Read the model definition and answer for the solid it produces. Units are mm, in the model's axes. Face numbers are marked on the shaded views. A direction names the side the tool comes from. Give positions to 0.01 mm unless a question says otherwise; leave off trailing zeros. Order: outer loops, then holes, each group sorted by start corner. A loop starts at its lowest first (then second) coordinate and runs counter-clockwise, first axis right, second up.
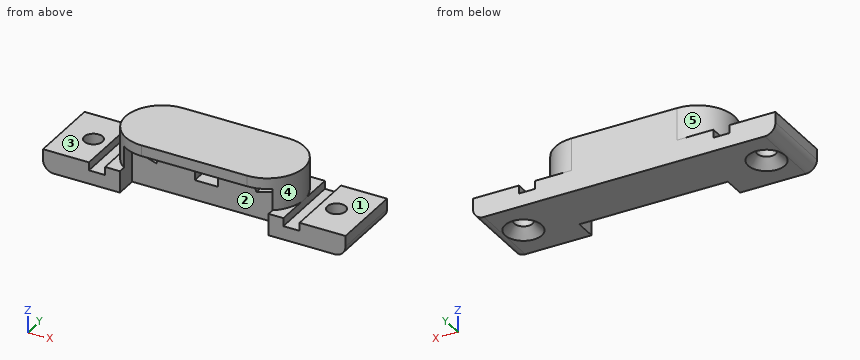
```python
from build123d import *

# Parameters (mm, degrees)
SKETCH_W        = 56
SKETCH_H        = 13.6
SKETCH_R        = 1.7
PAD_DEPTH       = 4
PAD001_DEPTH    = 6
SKETCH002_W     = 4.3
SKETCH002_H     = 1.7
POCKET_DEPTH    = 10
SKETCH003_W     = 27.5
SKETCH003_H     = 8.7
POCKET001_DEPTH = 4
SKETCH004_W     = 3
SKETCH004_H     = 1.5
POCKET002_DEPTH = 130.578947
CHAMFER_SIZE    = 1.7
CHAMFER001_SIZE = 1.7
FILLET_R        = 2
FILLET001_R     = 2


with BuildPart() as part:
    # Sketch → Pad (new body)
    with BuildSketch(Plane.XY):
        Rectangle(SKETCH_W, SKETCH_H)
        with Locations((-22.5, 0)):
            Circle(SKETCH_R, mode=Mode.SUBTRACT)
        with Locations((22.5, 0)):
            Circle(SKETCH_R, mode=Mode.SUBTRACT)
    extrude(amount=-PAD_DEPTH)

    # Sketch001 → Pad001 (new body)
    with BuildSketch(Plane.XY):
        with BuildLine():
            ThreePointArc((-9.75, 6.8), (-16.55, 0), (-9.75, -6.8))
            Line((-9.75, -6.8), (9.75, -6.8))
            ThreePointArc((9.75, -6.8), (16.55, 0), (9.75, 6.8))
            Line((-9.75, 6.8), (9.75, 6.8))
        make_face()
    extrude(amount=PAD001_DEPTH)

    # Sketch002 → Pocket (cut)
    with BuildSketch(Plane.XZ.offset(6.8)):
        Polygon((-12.857344, 3.612012), (-8.748385, 2.344555), (-9.249472, 0.720082), (-13.358432, 1.98754), align=None)
        with Locations((0, 0.5)):
            Rectangle(SKETCH002_W, SKETCH002_H)
        Polygon((8.748385, 2.344555), (12.857344, 3.612012), (13.358432, 1.98754), (9.249472, 0.720082), align=None)
    extrude(amount=-POCKET_DEPTH, mode=Mode.SUBTRACT)

    # Sketch003 → Pocket001 (cut)
    with BuildSketch(Plane.XZ.offset(6.8)):
        with Locations((0, -0.35)):
            Rectangle(SKETCH003_W, SKETCH003_H)
    extrude(amount=-POCKET001_DEPTH, mode=Mode.SUBTRACT)

    # Sketch004 → Pocket002 (cut, through all)
    with BuildSketch(Plane.XZ.offset(6.8)):
        with Locations((-18, -0.75)):
            Rectangle(SKETCH004_W, SKETCH004_H)
    pocket002 = extrude(amount=-POCKET002_DEPTH, mode=Mode.SUBTRACT)

    # Mirrored: Pocket002 across Sketch004 V_Axis
    add(pocket002.mirror(Plane(origin=(0, -6.8, 0), x_dir=(0, -1, 0), z_dir=(1, 0, 0))), mode=Mode.SUBTRACT)

    # Chamfer
    chamfer_edges = [part.edges().sort_by_distance(p)[0] for p in [
        (-24.2, 0, -4),
    ]]
    chamfer(chamfer_edges, length=CHAMFER_SIZE)

    # Chamfer001
    chamfer001_edges = [part.edges().sort_by_distance(p)[0] for p in [
        (20.8, 0, -4),
    ]]
    chamfer(chamfer001_edges, length=CHAMFER001_SIZE)

    # Fillet
    fillet_edges = [part.edges().sort_by_distance(p)[0] for p in [
        (-28, 0, -4),
    ]]
    fillet(fillet_edges, radius=FILLET_R)

    # Fillet001
    fillet001_edges = [part.edges().sort_by_distance(p)[0] for p in [
        (28, 0, -4),
    ]]
    fillet(fillet001_edges, radius=FILLET001_R)


solid = part.part
```
1) The part is cut by section C-C on y = 0. Count the separate pieces of the cut face and the enclosed holes in it, and give its area (3 significant figures).
Final values:
separate pieces: 3
enclosed holes: 3
area: 357 mm2
2) A tool of negligible diameter and unlimited length cuts with its end or side. For the marked faces 1, 2, 3, 4 and 5, from which of +Z, -Z, +X, -X, +Y, -Y can it reach the whole face along a straight path? Write none if from no direction.
Final values:
face 1: +Z, +X, +Y, -Y
face 2: -Z, -Y
face 3: +Z, -X, +Y, -Y
face 4: +Z, +X
face 5: +Z, -X
3) The part is cut by section A-A on z = -1. Determine the outline of the cut face in (x, y), and give its area (3 significant figures).
Final values:
outline: (-28, -6.8) - (-19.5, -6.8) - (-19.5, 6.8) - (-28, 6.8) - close; (-16.5, -6.8) - (-13.75, -6.8) - (-13.75, -2.8) - (13.75, -2.8) - (13.75, -6.8) - (16.5, -6.8) - (16.5, 6.8) - (-16.5, 6.8) - close; (19.5, -6.8) - (28, -6.8) - (28, 6.8) - (19.5, 6.8) - close; hole circle Ø3.4 at (-22.5, 0); hole circle Ø3.4 at (22.5, 0)
area: 552 mm2
4) The part is cut by section D-D on x = 1. Determine the outline of the cut face in (y, z).
Final values:
outline: (-6.8, 4) - (-2.8, 4) - (-2.8, 1.35) - (3.2, 1.35) - (3.2, -0.35) - (-2.8, -0.35) - (-2.8, -4) - (6.8, -4) - (6.8, 6) - (-6.8, 6) - close
5) Consider L1, parallel to Y at x = -22.5, z = -1.35; L2, parallel to Z at x = 18.5, y = -3; L3, parallel to Y at x = 5, z = 1.25. Determine where each line is inside the solid, lowest interval first.
Final values:
L1: y = -6.8 to -1.7, 1.7 to 6.8
L2: z = -4 to -1.5
L3: y = -2.8 to 6.8
6) Given pin 1 (0.8 mm diameter, centred on x = 15.5, y = -4.5, fed in from +Z); pin 2 (0.8 mm diameter, centred on y = 1, z = 0.5, fed in from -X); pin 3 (1.4 mm diameter, centred on x = 10, z = 3, fed in from -Y), each flat-ended and moving along its own axis, determine where each tip first touches the part or whether it passes through.
Final values:
pin 1: stops at z = 0
pin 2: stops at x = -16.52
pin 3: stops at y = -2.8
7) The part is cut by section B-B on x = 22.5. Determine the outline of the cut face in (y, z), and give its area (3 significant figures).
Final values:
outline: (-6.8, -4) - (-3.4, -4) - (-1.7, -2.3) - (-1.7, 0) - (-6.8, 0) - close; (1.7, -2.3) - (3.4, -4) - (6.8, -4) - (6.8, 0) - (1.7, 0) - close
area: 37.9 mm2
